from build123d import *

# Parameters (mm, degrees)
BOSS_EXTRUDE1_DEPTH = 3
CUT_EXTRUDE1_DEPTH  = 1.5
BOSS_EXTRUDE2_DEPTH = 3
FILLET1_R           = 10
SKETCH4_R           = 2.7
CUT_EXTRUDE2_DEPTH  = 193.117151759
SKETCH5_R           = 30
CUT_EXTRUDE3_DEPTH  = 193.117151759


with BuildPart() as part:
    # Sketch1 → Boss-Extrude1 (new body)
    with BuildSketch(Plane(origin=(0, 0, 0), x_dir=(0, 0, -1), z_dir=(1, 0, 0))):
        with BuildLine():
            Line((0, -18), (-120, -18))
            Line((-120, -18), (-120, -90))
            Line((-120, -90), (0, -90))
            ThreePointArc((0, -90), (63.639610307, -63.639610307), (90, 0))
            Line((90, 0), (90, 150))
            Line((90, 150), (18, 150))
            Line((18, 150), (18, 0))
            ThreePointArc((18, 0), (12.727922061, -12.727922061), (0, -18))
        make_face()
    extrude(amount=BOSS_EXTRUDE1_DEPTH)

    # Sketch2 → Cut-Extrude1 (cut)
    with BuildSketch(Plane(origin=(3, 0, 0), x_dir=(0, 0, -1), z_dir=(1, 0, 0))):
        with BuildLine():
            Line((0, -38), (-120, -38))
            Line((-120, -38), (-120, -36))
            Line((-120, -36), (0, -36))
            ThreePointArc((0, -36), (25.455844123, -25.455844123), (36, 0))
            Line((36, 0), (36, 150))
            Line((36, 150), (38, 150))
            Line((38, 150), (38, 0))
            ThreePointArc((38, 0), (26.870057685, -26.870057685), (0, -38))
        make_face()
        with BuildLine():
            Line((0, -80), (-120, -80))
            Line((-120, -80), (-120, -82))
            Line((-120, -82), (0, -82))
            ThreePointArc((0, -82), (57.982756057, -57.982756057), (82, 0))
            Line((82, 0), (82, 150))
            Line((82, 150), (80, 150))
            Line((80, 150), (80, 0))
            ThreePointArc((80, 0), (56.568542495, -56.568542495), (0, -80))
        make_face()
    extrude(amount=-CUT_EXTRUDE1_DEPTH, mode=Mode.SUBTRACT)

    # Sketch3 → Boss-Extrude2 (add)
    with BuildSketch(Plane(origin=(3, 0, 0), x_dir=(0, 0, -1), z_dir=(1, 0, 0))):
        with BuildLine():
            Line((-30, -90), (-30, -100))
            ThreePointArc((-30, -100), (-29.012585384, -94.647668653), (-26.180339887, -90))
            Line((-26.180339887, -90), (-30, -90))
        make_face()
        with BuildLine():
            ThreePointArc((-26.180339887, -90), (-29.012585384, -94.647668653), (-30, -100))
            Line((-30, -100), (0, -100))
            ThreePointArc((0, -100), (-0.987414616, -94.647668653), (-3.819660113, -90))
            Line((-3.819660113, -90), (-26.180339887, -90))
        make_face()
        with BuildLine():
            ThreePointArc((-3.819660113, -90), (-0.987414616, -94.647668653), (0, -100))
            Line((0, -100), (0, -90))
            Line((0, -90), (-3.819660113, -90))
        make_face()
        with BuildLine():
            Line((0, -100), (-30, -100))
            ThreePointArc((-30, -100), (-15, -115), (0, -100))
        make_face()
    extrude(amount=-BOSS_EXTRUDE2_DEPTH)

    # Fillet1
    fillet1_edges = [part.edges().sort_by_distance(p)[0] for p in [
        (1.5, -90, 0),
        (1.5, -90, 30),
    ]]
    fillet(fillet1_edges, radius=FILLET1_R - 0.0001)  # a hair under: the kernel refuses the full size

    # Sketch4 → Cut-Extrude2 (cut, through all)
    with BuildSketch(Plane(origin=(3, 0, 0), x_dir=(0, 0, -1), z_dir=(1, 0, 0))):
        with Locations((-15, -100)):
            Circle(SKETCH4_R)
    extrude(amount=-CUT_EXTRUDE2_DEPTH, mode=Mode.SUBTRACT)

    # Sketch5 → Cut-Extrude3 (cut, through all)
    with BuildSketch(Plane(origin=(3, 0, 0), x_dir=(0, 0, -1), z_dir=(1, 0, 0))):
        with Locations((-50.880906171, -2.772036536)):
            Circle(SKETCH5_R)
    extrude(amount=-CUT_EXTRUDE3_DEPTH, mode=Mode.SUBTRACT)


solid = part.part
Can you work these out from the model? Positions are in its coordinate system, mm. A direction names the side the tool comes from. Give positions to 0.01 mm unless a question says otherwise; leave off trailing zeros. Write each loop counter-clockwise with the first axis right and the second up, starting at its lowest first coordinate (ties: lowest second). Pieces come first, ordered by that corner, then holes. Notation, with made-up numbers: M 73.5,-27.5 L 81.5,-27.5 A9 ccw 81.5,-22.5 Z; hole C 17,88.25 d7. An arc over 180 degrees is marked long. Answer in a Markdown table with one row per item. Add a question column.
Item 1: We'd pull the mould along Z, two halves only. Please class faces 1 (the flat face through (3, -70, -47)), 2 (the cylindrical face through (1.52, -32.77, 51.32)), 3 (the cylindrical face through (1.48, -61.06, -66.12)): released by +Z, released by -Z, zero draft, split by the parting line, or undercut.
Item 2: Imagine slicing it at C-C, the plane y = -73.5. Write out the boundary of the cut face in (x, z).
Item 3: For pin 1 Ø0.8 at (x, z) = (2.5, 41.5) entering from -Y; pin 2 Ø1 at (x, z) = (2, -11) entering from +Y; pin 3 Ø1 at (x, y) = (2, -6.5) entering from -Z, each with a flat end and sliding along its axis, tell me the tip position at first contact or that it passes through.
Item 4: Please list where these lines run through material, in increasing order: L1, parallel to Y at x = 1.75, z = 90.5; L2, parallel to Y at x = 2.2, z = 15.
Item 5: Imagine slicing it at B-B, the plane y = 6. Write out the boundary of the cut face in (x, z).
Item 6: Imagine slicing it at A-A, the plane x = 2.5. State how many separate pieces and enclosed holes the cut face has, plus the area to 3 significant figures.
Item 7: On a 3-axis mill with a long thin cutter (end or side, diameter ignored), from which of +Z, -Z, +X, -X, +Y, -Y can I reach the whole of each face in a straight line? I mean faces 4 (the cylindrical face through (2.26, -26.573, -27.164)), 5 (the cylindrical face through (2, -115, 15)). Say none if no direction works.
Evaluation:
| question | item | result |
|---|---|---|
| 1 | face 1 | zero draft |
| 1 | face 2 | undercut |
| 1 | face 3 | released by -Z |
| 2 | outline | M 0,-51.94 L 3,-51.94 L 3,-36.36 L 1.5,-36.36 L 1.5,-31.59 L 3,-31.59 L 3,120 L 0,120 Z |
| 3 | pin 1 | stops at y = -90 |
| 3 | pin 2 | stops at y = -13.85 |
| 3 | pin 3 | stops at z = -89.8 |
| 4 | L1 | y = -90 to -82, -80 to -38, -36 to -18 |
| 4 | L2 | y = -115 to -102.7, -97.3 to -82, -80 to -38, -36 to -18 |
| 5 | outline | M 0,-90 L 3,-90 L 3,-82 L 1.5,-82 L 1.5,-80 L 3,-80 L 3,-38 L 1.5,-38 L 1.5,-36 L 3,-36 L 3,-18 L 0,-18 Z |
| 6 | separate pieces | 3 |
| 6 | enclosed holes | 1 |
| 6 | area | 24,200 mm² |
| 7 | face 4 | +X |
| 7 | face 5 | +X, -X, -Y |
